Autodesk Inventor part; units mm, degrees
ref_plane "YZ Plane" through (0, 0, 0) normal (1, 0, 0) x (0, 1, 0)
ref_plane "XZ Plane" through (0, 0, 0) normal (0, 1, 0) x (-1, 0, 0)
ref_plane "XY Plane" through (0, 0, 0) normal (0, 0, 1) x (1, 0, 0)
sketch "Sketch1" plane through (0, 0, 0) normal (0, 1, 0) x (-1, 0, 0)
  circle A0 centre (24.1, 110.65) radius 0.25
  circle A1 centre (-70.5, 110.65) radius 0.25
  circle A2 centre (-45.6, 89.15) radius 0.25
  circle A3 centre (0, 67.65) radius 0.25
  circle A4 centre (70.5, 42.15) radius 0.25
  circle A5 centre (32.15, 17.15) radius 0.25
  circle A6 centre (60.5, -17.65) radius 0.25
  circle A7 centre (-60.5, -17.65) radius 0.25
  circle A8 centre (24.1, -67.65) radius 0.25
  circle A9 centre (-70.5, -67.65) radius 0.25
  circle A10 centre (-45.6, -89.15) radius 0.25
  circle A11 centre (0, -110.65) radius 0.25
  circle A12 centre (-70.5, -110.65) radius 0.25
  circle A13 centre (70.5, -110.65) radius 0.25
  circle A14 centre (45.6, -89.15) radius 0.25
  circle A15 centre (-24.1, -67.65) radius 0.25
  circle A16 centre (70.5, -67.65) radius 0.25
  circle A17 centre (0, -17.65) radius 0.25
  circle A18 centre (-32.15, 17.15) radius 0.25
  circle A19 centre (-70.5, 42.15) radius 0.25
  circle A20 centre (-70.5, 67.65) radius 0.25
  circle A21 centre (70.5, 67.65) radius 0.25
  circle A22 centre (45.6, 89.15) radius 0.25
  circle A23 centre (-24.1, 110.65) radius 0.25
  circle A24 centre (70.5, 110.65) radius 0.25
  line L0 (75.5, -115.65) -> (75.5, -62.65)
  line L1 (75.5, -62.65) -> (65.5, -42.65)
  line L2 (65.5, -42.65) -> (65.5, 22.15)
  line L3 (65.5, 22.15) -> (75.5, 42.15)
  line L4 (75.5, 42.15) -> (75.5, 115.65)
  line L5 (75.5, 115.65) -> (30.5, 135.65)
  line L6 (30.5, 135.65) -> (-30.5, 135.65)
  line L7 (-30.5, 135.65) -> (-75.5, 115.65)
  line L8 (-75.5, 115.65) -> (-75.5, 42.15)
  line L9 (-75.5, 42.15) -> (-65.5, 22.15)
  line L10 (-65.5, 22.15) -> (-65.5, -42.65)
  line L11 (-65.5, -42.65) -> (-75.5, -62.65)
  line L12 (-75.5, -62.65) -> (-75.5, -115.65)
  line L13 (-75.5, -115.65) -> (-30.5, -135.65)
  line L14 (-30.5, -135.65) -> (30.5, -135.65)
  line L15 (30.5, -135.65) -> (75.5, -115.65)
  circle A25 centre (0, -110.65) radius 2
  circle A26 centre (70.5, -110.65) radius 2
  circle A27 centre (-70.5, -110.65) radius 2
  circle A28 centre (45.6, -89.15) radius 2
  circle A29 centre (-45.6, -89.15) radius 2
  circle A30 centre (70.5, -67.65) radius 2
  circle A31 centre (24.1, -67.65) radius 2
  circle A32 centre (-24.1, -67.65) radius 2
  circle A33 centre (-70.5, -67.65) radius 2
  circle A34 centre (60.5, -17.65) radius 2
  circle A35 centre (0, -17.65) radius 2
  circle A36 centre (-32.15, 17.15) radius 2
  circle A37 centre (-60.5, -17.65) radius 2
  circle A38 centre (32.15, 17.15) radius 2
  circle A39 centre (70.5, 42.15) radius 2
  circle A40 centre (-70.5, 42.15) radius 2
  circle A41 centre (-70.5, 67.65) radius 2
  circle A42 centre (0, 67.65) radius 2
  circle A43 centre (70.5, 67.65) radius 2
  circle A44 centre (45.6, 89.15) radius 2
  circle A45 centre (-45.6, 89.15) radius 2
  circle A46 centre (-70.5, 110.65) radius 2
  circle A47 centre (-24.1, 110.65) radius 2
  circle A48 centre (24.1, 110.65) radius 2
  circle A49 centre (70.5, 110.65) radius 2
  point P0 (0, 0)
  point P1 (0, 0)
  dimension "d0" = 4
  dimension "d1" = 4
  dimension "d2" = 4
  dimension "d3" = 4
  dimension "d4" = 4
  dimension "d5" = 4
  dimension "d6" = 4
  dimension "d7" = 4
  dimension "d8" = 4
  dimension "d9" = 4
  dimension "d10" = 4
  dimension "d11" = 4
  dimension "d12" = 4
  dimension "d13" = 4
  dimension "d14" = 4
  dimension "d15" = 4
  dimension "d16" = 4
  dimension "d17" = 4
  dimension "d18" = 4
  dimension "d19" = 4
  dimension "d20" = 4
  dimension "d21" = 4
  dimension "d22" = 4
  dimension "d23" = 4
  dimension "d24" = 4
extrude "Extrusion1" add sketch "Sketch1" along normal blind 2 contours L15 L14 L13 L12 L11 L10 L9 L8 L7 L6 L5 L4 L3 L2 L1 L0
sketch "Sketch2" plane through (0, 0, 0) normal (0, -1, 0) x (1, 0, 0)
  circle A0 centre (-70.5, 110.65) radius 2
  circle A1 centre (-24.1, 110.65) radius 2
  circle A2 centre (24.1, 110.65) radius 2
  circle A3 centre (70.5, 110.65) radius 2
  circle A4 centre (45.6, 89.15) radius 2
  circle A5 centre (-45.6, 89.15) radius 2
  circle A6 centre (-70.5, 67.65) radius 2
  circle A7 centre (0, 67.65) radius 2
  circle A8 centre (70.5, 67.65) radius 2
  circle A9 centre (70.5, 42.15) radius 2
  circle A10 centre (-70.5, 42.15) radius 2
  circle A11 centre (-32.15, 17.15) radius 2
  circle A12 centre (60.5, -17.65) radius 2
  circle A13 centre (32.15, 17.15) radius 2
  circle A14 centre (0, -17.65) radius 2
  circle A15 centre (-60.5, -17.65) radius 2
  circle A16 centre (70.5, -67.65) radius 2
  circle A17 centre (24.1, -67.65) radius 2
  circle A18 centre (-24.1, -67.65) radius 2
  circle A19 centre (-70.5, -67.65) radius 2
  circle A20 centre (45.6, -89.15) radius 2
  circle A21 centre (-45.6, -89.15) radius 2
  circle A22 centre (70.5, -110.65) radius 2
  circle A23 centre (-70.5, -110.65) radius 2
  circle A24 centre (0, -110.65) radius 2
  line L0 (65.5, 22.15) -> (75.5, 42.15)
  line L1 (75.5, 42.15) -> (75.5, 115.65)
  line L2 (75.5, 115.65) -> (30.5, 135.65)
  line L3 (30.5, 135.65) -> (-30.5, 135.65)
  line L4 (-30.5, 135.65) -> (-75.5, 115.65)
  line L5 (-75.5, 115.65) -> (-75.5, 42.15)
  line L6 (-75.5, 42.15) -> (-65.5, 22.15)
  line L7 (-65.5, 22.15) -> (-65.5, -42.65)
  line L8 (-65.5, -42.65) -> (-75.5, -62.65)
  line L9 (-75.5, -62.65) -> (-75.5, -115.65)
  line L10 (-75.5, -115.65) -> (-30.5, -135.65)
  line L11 (-30.5, -135.65) -> (30.5, -135.65)
  line L12 (30.5, -135.65) -> (75.5, -115.65)
  line L13 (75.5, -115.65) -> (75.5, -62.65)
  line L14 (75.5, -62.65) -> (65.5, -42.65)
  line L15 (65.5, -42.65) -> (65.5, 22.15)
  point P0 (0, 0)
extrude "Extrusion2" add sketch "Sketch2" along normal blind 1.3
sketch "Sketch3" plane through (0, -1.3, 0) normal (0, -1, 0) x (1, 0, 0)
  circle A0 centre (0, -110.65) radius 2
  circle A1 centre (-70.5, -110.65) radius 2
  circle A2 centre (70.5, -110.65) radius 2
  circle A3 centre (-45.6, -89.15) radius 2
  circle A4 centre (45.6, -89.15) radius 2
  circle A5 centre (-70.5, -67.65) radius 2
  circle A6 centre (-24.1, -67.65) radius 2
  circle A7 centre (24.1, -67.65) radius 2
  circle A8 centre (70.5, -67.65) radius 2
  circle A9 centre (-60.5, -17.65) radius 2
  circle A10 centre (0, -17.65) radius 2
  circle A11 centre (32.15, 17.15) radius 2
  circle A12 centre (60.5, -17.65) radius 2
  circle A13 centre (-32.15, 17.15) radius 2
  circle A14 centre (-70.5, 42.15) radius 2
  circle A15 centre (70.5, 42.15) radius 2
  circle A16 centre (70.5, 67.65) radius 2
  circle A17 centre (0, 67.65) radius 2
  circle A18 centre (-70.5, 67.65) radius 2
  circle A19 centre (-45.6, 89.15) radius 2
  circle A20 centre (45.6, 89.15) radius 2
  circle A21 centre (70.5, 110.65) radius 2
  circle A22 centre (24.1, 110.65) radius 2
  circle A23 centre (-24.1, 110.65) radius 2
  circle A24 centre (-70.5, 110.65) radius 2
  line L0 (65.5, 22.15) -> (75.5, 42.15)
  line L1 (75.5, 42.15) -> (75.5, 115.65)
  line L2 (75.5, 115.65) -> (30.5, 135.65)
  line L3 (30.5, 135.65) -> (-30.5, 135.65)
  line L4 (-30.5, 135.65) -> (-75.5, 115.65)
  line L5 (-75.5, 115.65) -> (-75.5, 42.15)
  line L6 (-75.5, 42.15) -> (-65.5, 22.15)
  line L7 (-65.5, 22.15) -> (-65.5, -42.65)
  line L8 (-65.5, -42.65) -> (-75.5, -62.65)
  line L9 (-75.5, -62.65) -> (-75.5, -115.65)
  line L10 (-75.5, -115.65) -> (-30.5, -135.65)
  line L11 (-30.5, -135.65) -> (30.5, -135.65)
  line L12 (30.5, -135.65) -> (75.5, -115.65)
  line L13 (75.5, -115.65) -> (75.5, -62.65)
  line L14 (75.5, -62.65) -> (65.5, -42.65)
  line L15 (65.5, -42.65) -> (65.5, 22.15)
  point P0 (0, 0)
extrude "Extrusion3" add sketch "Sketch3" along normal blind 8
sketch "Sketch4" plane through (0, 2, 0) normal (0, 1, 0) x (1, 0, 0)
  circle A0 centre (-32.15, -17.15) radius 2
  circle A1 centre (60.5, 17.65) radius 2
  circle A2 centre (32.15, -17.15) radius 2
  circle A3 centre (0, 17.65) radius 2
  circle A4 centre (-60.5, 17.65) radius 2
  point P0 (0, 0)
extrude "Extrusion4" add sketch "Sketch4" against normal blind 10
sketch "Sketch5" plane through (0, 2, 0) normal (0, 1, 0) x (1, 0, 0)
  circle A0 centre (-70.5, -67.65) radius 2
  circle A1 centre (0, -67.65) radius 2
  circle A2 centre (70.5, -67.65) radius 2
  circle A3 centre (24.1, 67.65) radius 2
  circle A4 centre (-24.1, 67.65) radius 2
  point P0 (0, 0)
extrude "Extrusion5" add sketch "Sketch5" against normal blind 10
properties part number "podvozek_komatex"
For this review, take the finished solid that the model builds, in its own axes (mm). A direction names the side the tool comes from. Round coordinates to 2 decimals unless told otherwise and drop trailing zeros. Write each loop counter-clockwise with the first axis right and the second up, starting at its lowest first coordinate (ties: lowest second). Pieces come first, ordered by that corner, then holes. Notation, with made-up numbers: (18, 21.25) - (74, 21.25) arc R12 cw to (74, 25.25) - close; hole circle Ø1 at (61, 75). An arc over 180 degrees is marked (long way). Answer as a JSON object with one key per item and string values.
1. Tool access review of faces 1 (the face through (-70.43, -3.57, -52.51)), 2 (the face through (70.43, -3.57, 32.01)), 3 (the face through (75.5, -4, 78)): name each direction out of +Z, -Z, +X, -X, +Y, -Y from which nothing blocks a thin tool from reaching the whole face with its end or side.
Response values:
{"face 1": "-X, +Y, -Y", "face 2": "+X, +Y, -Y", "face 3": "+Z, -Z, +X, +Y, -Y"}
2. For pin 1 Ø3 at (x, z) = (60.5, -18.5) entering from -Y; pin 2 Ø2 at (x, z) = (-32, 18) entering from -Y; pin 3 Ø1.5 at (y, z) = (-3, -42.5) entering from +X, all flat-tipped, find the tip position at first contact; note any pin that passes through.
Response values:
{"pin 1": "stops at y = -9.3", "pin 2": "stops at y = -8", "pin 3": "stops at x = 65.8"}
3. We need section A-A on y = -3.5. Count the separate pieces of the cut face and the enclosed holes in it, then the cut area to 3 significant figures.
Response values:
{"separate pieces": "1", "enclosed holes": "15", "area": "37,300 mm2"}
4. We need section C-C on x = 41. Give the boundary of the cut face in (y, z).
Response values:
{"outline": "(-9.3, -130.98) - (2, -130.98) - (2, 130.98) - (-9.3, 130.98) - close"}
5. Draft analysis for pull direction Z (two halves, no side actions). For faces 4 (the face through (-52.685, -3.571, 125.79)), 5 (the face through (-75.5, -4, -89)), 6 (the face through (-65.5, -4, -10)), 7 (the face through (-70.57, -3.57, 32.29)), state which applies: +Z half, -Z half, draft (parallel to the pull), parting line (faces both ways), or undercut.
Response values:
{"face 4": "+Z half", "face 5": "draft", "face 6": "undercut", "face 7": "undercut"}
6. We need section B-B on z = 3. Give the boundary of the cut face in (x, y).
Response values:
{"outline": "(-65.5, -9.3) - (65.5, -9.3) - (65.5, 2) - (-65.5, 2) - close"}
7. To check wall thickness, follow line 1 along X through (y, z) = (-0.95, -67.65); line 2 along X through (y, z) = (-1, 110.65); line 3 along X through (y, z) = (1, -90.5). State the ranges of each line that lie inside material, in increasing order.
Response values:
{"line 1": "x = -75.5 to -72.5, -68.5 to 68.5, 72.5 to 75.5", "line 2": "x = -75.5 to -72.5, -68.5 to -26.1, -22.1 to 22.1, 26.1 to 68.5, 72.5 to 75.5", "line 3": "x = -75.5 to -47.08, -44.12 to 44.12, 47.08 to 75.5"}
